Build history of the part. All positions in model axes, mm. A direction names the side the tool comes from. Give positions to 0.01 mm unless a question says otherwise; leave off trailing zeros. Write each loop counter-clockwise with the first axis right and the second up, starting at its lowest first coordinate (ties: lowest second). Pieces come first, ordered by that corner, then holes. Notation, with made-up numbers: (-20.5, -25.5) -> (31.5, -25.5) arc R23 cw to (31.5, 2.5) -> close; hole circle Ø7 at (51, 19). An arc over 180 degrees is marked (long way). One line per question, with ' | ' between items. Start each with the question number.
(1) Pull direction Z, two halves, no side cores. Call faces 3 (the flat face through (31, -61.6, 542)), 4 (the flat face through (31, 0, 542)), 5 (the flat face through (32, -31, 0)): released by +Z, released by -Z, zero draft, split by the parting line, or undercut.
(2) Band-saw the part on B-B, the plane z = 918.5. Give the cut face in (x, y), and give its area (3 significant figures).
(3) Band-saw the part on A-A, the plane y = -38. Give the cut face in (x, z), and give its area (3 significant figures).
(4) Drill centre lines: probe 1 along Z at (x, y) = (31.75, -62.7); probe 2 along Z at (x, y) = (20.5, -3.5); probe 3 along X at (y, z) = (-48, 425.5). Where is each one in solid material? Low to high. Write a range as from..to.
(5) Tool access for faces 1 (the flat face through (32, -31, 2)), 2 (the flat face through (31, -31, 1100)): list every direction of +Z, -Z, +X, -X, +Y, -Y with a clear straight run to the whole face (end or side of a thin tool).
from build123d import *

# Parameters (mm, degrees)
CROQUIS1_W              = 63.5
CROQUIS1_H              = 63.5
CROQUIS1_W_2            = 59.7
CROQUIS1_H_2            = 59.7
SALIENTE_EXTRUIR1_DEPTH = 1100
CROQUIS2_W              = 59.7
CROQUIS2_H              = 59.7
SALIENTE_EXTRUIR2_DEPTH = 2
CROQUIS3_W              = 59.7
CROQUIS3_H              = 59.7
SALIENTE_EXTRUIR3_DEPTH = 2
CROQUIS4_R              = 7.14375
CORTAR_EXTRUIR1_DEPTH   = 120


with BuildPart() as part:
    # Croquis1 → Saliente-Extruir1 (new body)
    with BuildSketch(Plane.XY):
        with Locations((31.75, -31.75)):
            Rectangle(CROQUIS1_W, CROQUIS1_H)
        with Locations((31.75, -31.75)):
            Rectangle(CROQUIS1_W_2, CROQUIS1_H_2, mode=Mode.SUBTRACT)
    extrude(amount=SALIENTE_EXTRUIR1_DEPTH)

    # Croquis2 → Saliente-Extruir2 (add)
    with BuildSketch(Plane.XY.offset(1100)):
        with Locations((31.75, -31.75)):
            Rectangle(CROQUIS2_W, CROQUIS2_H)
    extrude(amount=-SALIENTE_EXTRUIR2_DEPTH)

    # Croquis3 → Saliente-Extruir3 (add)
    with BuildSketch(Plane(origin=(0, 0, 0), x_dir=(-1, 0, 0), z_dir=(0, 0, -1))):
        with Locations((-31.75, -31.75)):
            Rectangle(CROQUIS3_W, CROQUIS3_H)
    extrude(amount=-SALIENTE_EXTRUIR3_DEPTH)

    # Croquis4 → Cortar-Extruir1 (cut)
    with BuildSketch(Plane(origin=(0, 0, 0), x_dir=(1, 0, 0), z_dir=(0, 1, 0))):
        with Locations((31.75, -160)):
            Circle(CROQUIS4_R)
        with Locations((31.75, -745)):
            Circle(CROQUIS4_R)
    extrude(amount=-CORTAR_EXTRUIR1_DEPTH, mode=Mode.SUBTRACT)


solid = part.part
Results:
1) face 3: undercut | face 4: zero draft | face 5: released by -Z
2) outline: (0, -63.5) -> (63.5, -63.5) -> (63.5, 0) -> (0, 0) -> close; hole (1.9, -61.6) -> (61.6, -61.6) -> (61.6, -1.9) -> (1.9, -1.9) -> close | area: 468 mm²
3) outline: (0, 0) -> (63.5, 0) -> (63.5, 1100) -> (0, 1100) -> close; hole (1.9, 2) -> (61.6, 2) -> (61.6, 1098) -> (1.9, 1098) -> close | area: 4,420 mm²
4) probe 1: z = 0..152.86, 167.14..737.86, 752.14..1100 | probe 2: z = 0..2, 1098..1100 | probe 3: x = 0..1.9, 61.6..63.5
5) face 1: none | face 2: +Z, +X, -X, +Y, -Y
